Geometry: final body of the model. Coordinates: model frame, mm. Give positions to 0.01 mm unless a question says otherwise; leave off trailing zeros. Order: outer loops, then holes, each group sorted by start corner. A loop starts at its lowest first (then second) coordinate and runs counter-clockwise, first axis right, second up. Notation, with made-up numbers: (-33, 28) -> (-12, 28) arc R33 ccw to (-12, 60) -> close; hole circle Ø11 at (76.25, 62). An arc over 180 degrees is marked (long way). Write item = value, one per line.
```python
from build123d import *

# Parameters (mm, degrees)
F0_R            = 2.5
F1_DEPTH        = 11
F2_DEPTH        = 7
F2_COPIES_COUNT = 40


# Not quite as in the source:
# - a pattern or mirror of a feature is missing from the dataset's text; its kind, count and spacing are read off the source's solid


with BuildPart() as f1:
    # F0 (on Front) → F1 (new body)
    with BuildSketch(Plane.XZ):
        with BuildLine():
            ThreePointArc((-0.7821723252, 4.938441703), (-3.2472402417, -3.802029828), (5, 0))
            ThreePointArc((5, 0), (3.5355339059, 3.5355339059), (0, 5))
            ThreePointArc((0, 5), (-0.3922954786, 4.9845866687), (-0.7821723252, 4.938441703))
        make_face()
        Circle(F0_R, mode=Mode.SUBTRACT)
    extrude(amount=F1_DEPTH)

    # F0 (on Front) → F2 (join)
    with BuildSketch(Plane.XZ):
        with BuildLine():
            ThreePointArc((-0.7821723252, 4.938441703), (-0.3922954786, 4.9845866687), (0, 5))
            Line((0, 5), (-0.4315250265, 5.4830453355))
            Line((-0.4315250265, 5.4830453355), (-0.7821723252, 4.938441703))
        make_face()
    f2 = extrude(amount=F2_DEPTH)

    # F2_copies: F2 ×40 about axis
    f2_copies_axis = Axis((0, 0, 0), (0, 1, 0))
    for i in range(1, F2_COPIES_COUNT):
        add(f2.rotate(f2_copies_axis, i * 360 / F2_COPIES_COUNT))

    # F3 (on Top) → F4 (revolve, cut)
    with BuildSketch(Plane.XY):
        Polygon((8, 0), (5, 0), (7, -2), (7, -5), (5, -7), (8, -7), align=None)
    revolve(axis=Axis((0, -7.7233230695, 0), (0, -1, 0)), mode=Mode.SUBTRACT)


solid = f1.part
```
1) First-contact query: P1, Ø1.5, axis at y = -8.5, z = -0.5, coming from the -X side. Flat tip, straight axial feed; report the tip coordinate or a pass-through.
Check sheet entries:
P1 = -5
2) Mould query, pull axis X, two halves, no side actions, for faces 1 (the face through (2, -11, -2)), 2 (the face through (-0.54, -5.42, -2.44)). Classes: +X half, -X half, draft (parallel to the pull), parting line (faces both ways), or undercut.
Check sheet entries:
face_1 = draft
face_2 = undercut
3) Line query: line 1 (Z direction, x = 0, y = -7.5); line 2 (Z direction, x = -1.25, y = -1.25); line 3 (X direction, y = -3.5, z = -2.75). Output: solid intervals per line, ascending. Write a range as from..to.
Check sheet entries:
line_1 = -5..-2.5, 2.5..5
line_2 = -5.32..-2.17, 2.17..5.32
line_3 = -4.64..4.64
4) Section query A-A (y = -10). Output: boundary loops of the cut face in (x, z), plus the area to 3 significant figures.
Check sheet entries:
outline = circle Ø10 at (0, 0); hole circle Ø5 at (0, 0)
area = 58.9 mm²
